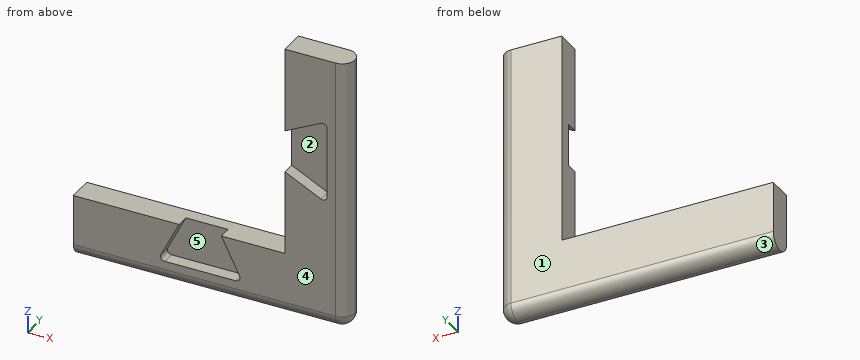
Autodesk Inventor part; units mm, degrees
ref_plane "YZ Plane" through (0, 0, 0) normal (1, 0, 0) x (0, 1, 0)
ref_plane "XZ Plane" through (0, 0, 0) normal (0, 1, 0) x (-1, 0, 0)
ref_plane "XY Plane" through (0, 0, 0) normal (0, 0, 1) x (1, 0, 0)
sketch "Sketch1" plane through (0, 0, 0) normal (0, 1, 0) x (-1, 0, 0)
  line L0 (100, -50) -> (-100, -50)
  line L1 (-100, -50) -> (-100, 50)
  line L2 (-100, 50) -> (100, 50)
  line L3 (100, 50) -> (100, -50)
  line L4 (100, -50) -> (-100, 50) construction
  line L5 (-100, -50) -> (100, 50) construction
  line L6 (-40, -30) -> (-80, -30)
  line L7 (-50, -50) -> (-70, -50)
  line L8 (-40, -30) -> (-50, -50)
  line L9 (-80, -30) -> (-70, -50)
  line L10 (80, -30) -> (40, -30)
  line L11 (70, -50) -> (50, -50)
  line L12 (80, -30) -> (70, -50)
  line L13 (40, -30) -> (50, -50)
  line L14 (-100, -10) -> (-100, 10)
  line L15 (-80, -20) -> (-80, 20)
  line L16 (-80, -20) -> (-100, -10)
  line L17 (-80, 20) -> (-100, 10)
  line L18 (-100, -50) -> (-130, -50)
  line L19 (-130, -50) -> (-130, 50)
  line L20 (-130, 50) -> (-100, 50)
  line L21 (-100, 50) -> (-100, -50)
  line L22 (-130, -50) -> (0, -50)
  line L23 (0, -50) -> (0, -80)
  line L24 (0, -80) -> (-130, -80)
  line L25 (-130, -80) -> (-130, -50)
  line L26 (-40, -70) -> (-80, -70)
  line L27 (-40, -70) -> (-50, -50)
  line L28 (-80, -70) -> (-70, -50)
  line L29 (-120, -20) -> (-120, 20)
  line L30 (-120, -20) -> (-100, -10)
  line L31 (-120, 20) -> (-100, 10)
  point P0 (0, 0)
  point P1 (-100, 10)
  point P2 (-100, -10)
  point P3 (-70, -50)
  point P4 (-50, -50)
  point P5 (70, -50)
  point P6 (0, 0)
  point P7 (0, 0)
  point P8 (0, -50)
  dimension "d72" = 200
  dimension "d73" = 100
  dimension "d78" = 20
  dimension "d79" = 40
  dimension "d80" = 20
  dimension "d81" = 10
  dimension "d82" = 20
  dimension "d83" = 40
  dimension "d84" = 20
  dimension "d85" = 10
  dimension "d86" = 120
  dimension "d87" = 30
  dimension "d88" = 0
  dimension "d89" = 0
  dimension "d90" = 40
  dimension "d91" = 20
  dimension "d92" = 20
  dimension "d93" = 10
  dimension "d94" = 40
  dimension "d95" = 0
  dimension "d114" = 30
  dimension "d115" = 130
  dimension "d116" = 30
extrude "Extrusion24" add sketch "Sketch1" along normal blind 12 contours L1 L31 L29 L30 L18 L19 L20 | L23 L24 L25 L18 L0 L28 L26 L27 | L1 L30 L29 L31 | L27 L26 L28 L0
extrude "Extrusion25" cut sketch "Sketch1" along normal blind 6 contours L1 L30 L29 L31 | L27 L26 L28 L0
fillet "Fillet12" radius 2 4 edges at (120, 3, 20) (120, 3, -20) (80, 3, -70) (40, 3, -70)
fillet "Fillet13" radius 6 5 edges at (130, 0, -15) (130, 12, -15) (65, 12, -80) (65, 0, -80) (130, 6, -80)
properties part number "Test2_3DPrint"
Read the model definition and answer for the solid it produces. Units are mm, in the model's axes. Face numbers are marked on the shaded views. A direction names the side the tool comes from. Give positions to 0.01 mm unless a question says otherwise; leave off trailing zeros. Write each loop counter-clockwise with the first axis right and the second up, starting at its lowest first coordinate (ties: lowest second). Pieces come first, ordered by that corner, then holes. Notation, with made-up numbers: (78.5, 31.25) - (96.5, 31.25) arc R28 ccw to (96.5, 52.25) - close; hole circle Ø4 at (58, 24). An arc over 180 degrees is marked (long way). Answer in a Markdown table with one row per item. Add a question column.
Item 1: Flat-ended cylindrical pins translate along their axes: P1, Ø10, axis at x = 28.5, z = -55.5, coming from the -Y side; P2, Ø6.5, axis at x = 55, y = 4.5, coming from the +Z side; P3, Ø6, axis at y = 8.5, z = 14, coming from the -X side; P4, Ø6, axis at y = 2, z = -65, coming from the +X side. Find the tip coordinate at first contact, or state that the pin passes through.
Item 2: A tool of negligible diameter and unlimited length cuts with its end or side. For the marked faces 4 and 5, from which of +Z, -Z, +X, -X, +Y, -Y can it reach the whole face along a straight path? Write none if from no direction.
Item 3: Find the intervals of material crossed by L1, parallel to Y at x = 59, z = -66; L2, parallel to X at y = 1.5, z = -59; L3, parallel to Z at x = 97.5, y = 6, in increasing order.
Item 4: Section C-C, the plane y = 9.75 is taken. Write down the section's boundary in (x, z).
Item 5: Determine the mould class of the marked faces 1, 2 and 3 for opening direction Z: pulls with the +Z half, pulls with the -Z half, needs draft (parallel to the pull), parting line crosses it, or undercut.
Recorded:
| question | item | result |
|---|---|---|
| 1 | P1 | stops at y = 0 |
| 1 | P2 | stops at z = -50 |
| 1 | P3 | stops at x = 100 |
| 1 | P4 | stops at x = 129.92 |
| 2 | face 4 | +Z, -Z, +X, -X, -Y |
| 2 | face 5 | -Y |
| 3 | L1 | y = 6 to 12 |
| 3 | L2 | x = 0 to 45.5, 74.5 to 127.97 |
| 3 | L3 | z = -80 to -50 |
| 4 | outline | (0, -78.68) - (124, -78.68) arc R4.68 ccw to (128.68, -74) - (128.68, 50) - (100, 50) - (100, -50) - (0, -50) - close |
| 5 | face 1 | needs draft |
| 5 | face 2 | undercut |
| 5 | face 3 | pulls with the -Z half |
